Can you work these out from the model? Positions are in its coordinate system, mm. A direction names the side the tool comes from. Give positions to 0.01 mm unless a question says otherwise; leave off trailing zeros. Write each loop counter-clockwise with the first axis right and the second up, starting at its lowest first coordinate (ties: lowest second). Pieces come first, ordered by that corner, then holes.
1. Suppose I cut it at A-A (x = 66). Please give me the cut outline in (y, z), and give its area (3 significant figures).
2. Thinking about a two-plate mould opening in X: for faces 1 (the flat face through (-1, -12.7, 9)), 2 (the cylindrical face through (-1.05, 1.67, 9.66)), 3 (the flat face through (82.55, -9, 9)), 4 (the flat face through (-82.55, 0, 9)), which applies, pulls with the +X half, pulls with the -X half, needs draft (parallel to the pull), parting line crosses it, or undercut?
3. I'm going to push flat-ended pins straight in: pin 1 (3 mm diameter, centred on y = -0.5, z = 12.5, fed in from +X); pin 2 (13 mm diameter, centred on x = -6.35, y = 0, fed in from -Z). Where does each tip first touch, or does it pass through?
4. On a 3-axis mill with a long thin cutter (end or side, diameter ignored), from which of +Z, -Z, +X, -X, +Y, -Y can I reach the whole of each face in a straight line? I mean faces 5 (the flat face through (63.5, 0, 10)), 6 (the cylindrical face through (-52.02, -2.13, 9.66)). Say none if no direction works.
5. Suppose I cut it at D-D (x = -57.15). Please give me the cut outline in (y, z).
6. Suppose I cut it at C-C (y = 0). Please give me the cut outline in (x, z).
7. If I drill on probe 1 along Y at (x, z) = (44.45, 10.5); probe 2 along Y at (x, z) = (-60, 6.5); probe 3 along X at (y, z) = (-3.5, 18), over which ranges is the centre line in solid material (lowest first)?
8. Suppose I cut it at B-B (z = 9.5). Please give me the cut outline in (x, y), and give its area (3 significant figures).
```python
from build123d import *

# Parameters (mm, degrees)
F0_W     = 165.1
F0_H     = 25.4
F1_DEPTH = 19.05
F2_W     = 19.05
F2_H     = 9.525
F3_DEPTH = 19.051
F4_R     = 5.55625
F5_DEPTH = 19.051


with BuildPart() as f1:
    # F0 (on Top) → F1 (new body)
    with BuildSketch(Plane.XY):
        Rectangle(F0_W, F0_H)
    extrude(amount=F1_DEPTH)

    # F2 (on face) → F3 (cut, through all)
    with BuildSketch(Plane.XY.offset(19.05)):
        with Locations((73.025, 0)):
            Rectangle(F2_W, F2_H)
    extrude(amount=-F3_DEPTH, mode=Mode.SUBTRACT)

    # F4 (on face) → F5 (cut, through all)
    with BuildSketch(Plane.XY.offset(19.05)):
        with Locations((-57.15, 0)):
            Circle(F4_R)
        with Locations((-6.35, 0)):
            Circle(F4_R)
        with Locations((44.45, 0)):
            Circle(F4_R)
    extrude(amount=-F5_DEPTH, mode=Mode.SUBTRACT)


solid = f1.part
```
Checks:
1. outline: (-12.7, 0) - (-4.76, 0) - (-4.76, 19.05) - (-12.7, 19.05) - close; (4.76, 0) - (12.7, 0) - (12.7, 19.05) - (4.76, 19.05) - close
1. area: 302 mm2
2. face 1: needs draft
2. face 2: undercut
2. face 3: pulls with the +X half
2. face 4: pulls with the -X half
3. pin 1: stops at x = 63.5
3. pin 2: stops at z = 0
4. face 5: +Z, -Z, +X
4. face 6: +Z, -Z
5. outline: (-12.7, 0) - (-5.56, 0) - (-5.56, 19.05) - (-12.7, 19.05) - close; (5.56, 0) - (12.7, 0) - (12.7, 19.05) - (5.56, 19.05) - close
6. outline: (-82.55, 0) - (-62.71, 0) - (-62.71, 19.05) - (-82.55, 19.05) - close; (-51.59, 0) - (-11.91, 0) - (-11.91, 19.05) - (-51.59, 19.05) - close; (-0.79, 0) - (38.89, 0) - (38.89, 19.05) - (-0.79, 19.05) - close; (50.01, 0) - (63.5, 0) - (63.5, 19.05) - (50.01, 19.05) - close
7. probe 1: y = -12.7 to -5.56, 5.56 to 12.7
7. probe 2: y = -12.7 to -4.77, 4.77 to 12.7
7. probe 3: x = -82.55 to -61.47, -52.83 to -10.67, -2.03 to 40.13, 48.77 to 63.5
8. outline: (-82.55, -12.7) - (82.55, -12.7) - (82.55, -4.76) - (63.5, -4.76) - (63.5, 4.76) - (82.55, 4.76) - (82.55, 12.7) - (-82.55, 12.7) - close; hole circle Ø11.11 at (-57.15, 0); hole circle Ø11.11 at (-6.35, 0); hole circle Ø11.11 at (44.45, 0)
8. area: 3,720 mm2
